```python
from build123d import *

# Parameters (mm, degrees)
SKETCH1_W           = 58
SKETCH1_H           = 95
BOSS_EXTRUDE1_DEPTH = 4
SKETCH2_R           = 4
SKETCH2_R_2         = 1.45
BOSS_EXTRUDE2_DEPTH = 7
FILLET1_R           = 5
CUT_EXTRUDE1_REACH  = 58.73
SKETCH3_R           = 2.4


with BuildPart() as part:
    # Sketch1 → Boss-Extrude1 (new body)
    with BuildSketch(Plane(origin=(0, 0, 0), x_dir=(1, 0, 0), z_dir=(0, 1, 0))):
        Rectangle(SKETCH1_W, SKETCH1_H)
    extrude(amount=BOSS_EXTRUDE1_DEPTH)

    # Sketch2 → Boss-Extrude2 (add)
    # profile 1 of 6: a face of its own
    with BuildSketch(Plane(origin=(0, 4, 0), x_dir=(1, 0, 0), z_dir=(0, 1, 0))):
        with Locations(Location((-24, 40.1, 0), (0, 0, 270))):
            Circle(SKETCH2_R)
        with Locations(Location((-24, 40.1, 0), (0, 0, 270))):
            Circle(SKETCH2_R_2, mode=Mode.SUBTRACT)
    # profile 2 of 6: a face of its own
    with BuildSketch(Plane(origin=(0, 4, 0), x_dir=(1, 0, 0), z_dir=(0, 1, 0))):
        with Locations(Location((24.25, 38.85, 0), (0, 0, 270))):
            Circle(SKETCH2_R)
        with Locations(Location((24.25, 38.85, 0), (0, 0, 270))):
            Circle(SKETCH2_R_2, mode=Mode.SUBTRACT)
    # profile 3 of 6: a face of its own
    with BuildSketch(Plane(origin=(0, 4, 0), x_dir=(1, 0, 0), z_dir=(0, 1, 0))):
        with Locations(Location((-18.9, -11.9, 0), (0, 0, 270))):
            Circle(SKETCH2_R)
        with Locations(Location((-18.9, -11.9, 0), (0, 0, 270))):
            Circle(SKETCH2_R_2, mode=Mode.SUBTRACT)
    # profile 4 of 6: a face of its own
    with BuildSketch(Plane(origin=(0, 4, 0), x_dir=(1, 0, 0), z_dir=(0, 1, 0))):
        with Locations(Location((9.1, -11.9, 0), (0, 0, 270))):
            Circle(SKETCH2_R)
        with Locations(Location((9.1, -11.9, 0), (0, 0, 270))):
            Circle(SKETCH2_R_2, mode=Mode.SUBTRACT)
    # profile 5 of 6: a face of its own
    with BuildSketch(Plane(origin=(0, 4, 0), x_dir=(1, 0, 0), z_dir=(0, 1, 0))):
        with Locations(Location((-24, -42.4, 0), (0, 0, 270))):
            Circle(SKETCH2_R)
        with Locations(Location((-24, -42.4, 0), (0, 0, 270))):
            Circle(SKETCH2_R_2, mode=Mode.SUBTRACT)
    # profile 6 of 6: a face of its own
    with BuildSketch(Plane(origin=(0, 4, 0), x_dir=(1, 0, 0), z_dir=(0, 1, 0))):
        with Locations(Location((24.3, -36.1, 0), (0, 0, 270))):
            Circle(SKETCH2_R)
        with Locations(Location((24.3, -36.1, 0), (0, 0, 270))):
            Circle(SKETCH2_R_2, mode=Mode.SUBTRACT)
    extrude(amount=BOSS_EXTRUDE2_DEPTH)

    # Fillet1
    fillet1_edges = [part.edges().sort_by_distance(p)[0] for p in [
        (29, 2, 47.5),
        (-29, 2, 47.5),
        (-29, 2, -47.5),
        (29, 2, -47.5),
    ]]
    fillet(fillet1_edges, radius=FILLET1_R)

    # Sketch3 → Cut-Extrude1 (cut, up to next)
    with BuildSketch(Plane(origin=(0, 0, 0), x_dir=(1, 0, 0), z_dir=(0, 1, 0)), mode=Mode.PRIVATE) as cut_extrude1_sk1:
        with Locations(Location((-12, 20, 0), (0, 0, 270))):
            Circle(SKETCH3_R)
    cut_extrude1_tool1 = extrude(cut_extrude1_sk1.sketch, amount=CUT_EXTRUDE1_REACH, mode=Mode.PRIVATE) & part.part
    # Sketch3 → Cut-Extrude1 (cut, up to next)
    with BuildSketch(Plane(origin=(0, 0, 0), x_dir=(1, 0, 0), z_dir=(0, 1, 0)), mode=Mode.PRIVATE) as cut_extrude1_sk2:
        with Locations(Location((12, 20, 0), (0, 0, 270))):
            Circle(SKETCH3_R)
    cut_extrude1_tool2 = extrude(cut_extrude1_sk2.sketch, amount=CUT_EXTRUDE1_REACH, mode=Mode.PRIVATE) & part.part
    # Sketch3 → Cut-Extrude1 (cut, up to next)
    with BuildSketch(Plane(origin=(0, 0, 0), x_dir=(1, 0, 0), z_dir=(0, 1, 0)), mode=Mode.PRIVATE) as cut_extrude1_sk3:
        with Locations(Location((-12, -20, 0), (0, 0, 270))):
            Circle(SKETCH3_R)
    cut_extrude1_tool3 = extrude(cut_extrude1_sk3.sketch, amount=CUT_EXTRUDE1_REACH, mode=Mode.PRIVATE) & part.part
    # Sketch3 → Cut-Extrude1 (cut, up to next)
    with BuildSketch(Plane(origin=(0, 0, 0), x_dir=(1, 0, 0), z_dir=(0, 1, 0)), mode=Mode.PRIVATE) as cut_extrude1_sk4:
        with Locations(Location((12, -20, 0), (0, 0, 270))):
            Circle(SKETCH3_R)
    cut_extrude1_tool4 = extrude(cut_extrude1_sk4.sketch, amount=CUT_EXTRUDE1_REACH, mode=Mode.PRIVATE) & part.part
    add(cut_extrude1_tool1.solids().sort_by_distance((-12, 0, -20))[0], mode=Mode.SUBTRACT)
    add(cut_extrude1_tool2.solids().sort_by_distance((12, 0, -20))[0], mode=Mode.SUBTRACT)
    add(cut_extrude1_tool3.solids().sort_by_distance((-12, 0, 20))[0], mode=Mode.SUBTRACT)
    add(cut_extrude1_tool4.solids().sort_by_distance((12, 0, 20))[0], mode=Mode.SUBTRACT)


solid = part.part
```
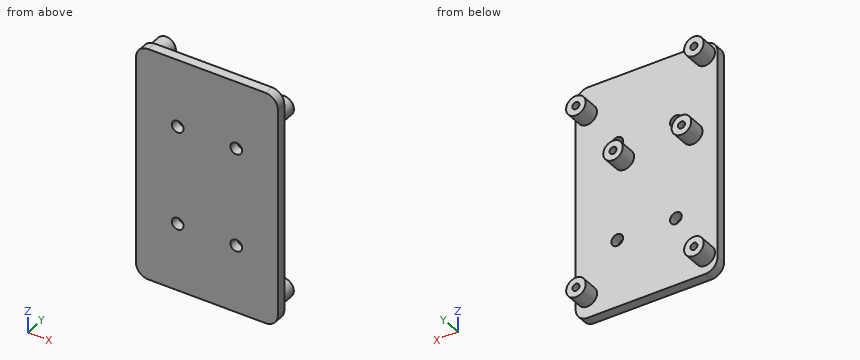
For this review, take the finished solid that the model builds, in its own axes (mm). Give positions to 0.01 mm unless a question says otherwise; leave off trailing zeros. Write each loop counter-clockwise with the first axis right and the second up, starting at its lowest first coordinate (ties: lowest second). Pieces come first, ordered by that corner, then holes.
Item 1: Wall thickness on probe 1 along X at (y, z) = (8.5, 11.9); probe 2 along Z at (x, y) = (-12, 2.4); probe 3 along X at (y, z) = (8.75, 36.1): over which ranges is each line inside the solid? List them lowest first.
Item 2: Take a section at B-B (x = -12). Give the boundary of the cut face in (y, z).
Item 3: Take a section at A-A (y = 8.75). Give the number of separate pieces and of enclosed holes in the cut face, and give its area (3 significant figures).
Item 4: Take a section at D-D (z = 33.5). Give the boundary of the cut face in (x, y).
Item 5: Take a section at C-C (y = 1). Give the boundary of the cut face in (x, z).
Item 6: Insertion check: P1, Ø6, axis at x = -14, z = 3, coming from the +Y side; P2, Ø3, axis at y = 6.5, z = 0.5, coming from the +X side; P3, Ø3, axis at y = 6.5, z = 12, coming from the -X side. Each pin has a flat end and moves straight along its axis. Give the tip position at first contact, or say it passes through.
Established:
1. probe 1: x = -22.9 to -20.35, -17.45 to -14.9, 5.1 to 7.65, 10.55 to 13.1
1. probe 2: z = -47.5 to -22.4, -17.6 to 17.6, 22.4 to 47.5
1. probe 3: x = 20.3 to 22.85, 25.75 to 28.3
2. outline: (0, -47.5) - (4, -47.5) - (4, -22.4) - (0, -22.4) - close; (0, -17.6) - (4, -17.6) - (4, 17.6) - (0, 17.6) - close; (0, 22.4) - (4, 22.4) - (4, 47.5) - (0, 47.5) - close
3. separate pieces: 6
3. enclosed holes: 6
3. area: 262 mm2
4. outline: (-29, 0) - (29, 0) - (29, 4) - (27.34, 4) - (27.34, 11) - (21.26, 11) - (21.26, 4) - (-29, 4) - close
5. outline: (-29, -42.5) arc R5 ccw to (-24, -47.5) - (24, -47.5) arc R5 ccw to (29, -42.5) - (29, 42.5) arc R5 ccw to (24, 47.5) - (-24, 47.5) arc R5 ccw to (-29, 42.5) - close; hole circle Ø4.8 at (-12, -20); hole circle Ø4.8 at (-12, 20); hole circle Ø4.8 at (12, -20); hole circle Ø4.8 at (12, 20)
6. P1: stops at y = 4
6. P2: passes through
6. P3: stops at x = -22.9
